The model under review builds one solid part; all positions refer to its coordinate system, in mm. A direction names the side the tool comes from. Give positions to 0.01 mm unless a question says otherwise; leave off trailing zeros. Order: outer loops, then holes, each group sorted by start corner. A loop starts at its lowest first (then second) coordinate and runs counter-clockwise, first axis right, second up.
```python
from build123d import *

# Parameters (mm, degrees)
F1_DEPTH  = 17.5
F2_R      = 2.25021
F2_R_2    = 2.117892
F2_R_3    = 2.141219
F2_R_4    = 1.925027
F2_R_5    = 3.371511
F2_R_6    = 3.105781
F2_R_7    = 1.98861
F2_R_8    = 1.899979
F2_R_9    = 1.912547
F3_DEPTH  = 40
F4_R      = 2.117892
F4_R_2    = 2.25021
F5_DEPTH  = 5
F6_R      = 2.141219
F6_R_2    = 1.925027
F7_DEPTH  = 3
F9_DEPTH  = 3
F10_W     = 16.805832
F10_H     = 44.291496
F10_R     = 3.105781
F10_R_2   = 3.371511
F11_DEPTH = 2


with BuildPart() as f1:
    # F0 (on Front) → F1 (new body)
    with BuildSketch(Plane.XZ):
        Polygon((-29.036315, 123.591392), (-62.036315, 123.591392), (-62.036315, 112.341392), (-79.036315, 112.341392), (-79.036315, 101.091392), (-95.036315, 101.091392), (-95.036315, 56.091392), (-79.036315, 56.091392), (-79.313149, 44.841392), (-62.036315, 44.841392), (-62.036315, 33.591392), (-29.036315, 33.591392), (-29.036315, 58.591392), (-35.036315, 58.591392), (-35.036315, 98.591392), (-29.036315, 98.591392), align=None)
    extrude(amount=F1_DEPTH)

    # F2 (on face) → F3 (cut)
    with BuildSketch(Plane(origin=(-95.036315, 0, 0), x_dir=(0, -1, 0), z_dir=(-1, 0, 0))):
        with Locations((13.294209, 118.739031)):
            Circle(F2_R)
        with Locations((4.177382, 118.739031)):
            Circle(F2_R_2)
        with Locations((4.177382, 106.985271)):
            Circle(F2_R_3)
        with Locations((13.294209, 106.985271)):
            Circle(F2_R_4)
        with Locations((4.177382, 95.644102)):
            Circle(F2_R_5)
        with Locations((4.177382, 84.471688)):
            Circle(F2_R_6)
        with Locations((4.177382, 39.11674)):
            Circle(F2_R_7)
        with Locations((8.744364, 39.11674)):
            Circle(F2_R_8)
        with Locations((13.294209, 39.11674)):
            Circle(F2_R_9)
    extrude(amount=-F3_DEPTH, mode=Mode.SUBTRACT)

    # F4 (on face) → F5 (cut)
    with BuildSketch(Plane(origin=(-62.036315, 0, 0), x_dir=(0, -1, 0), z_dir=(-1, 0, 0))):
        with BuildLine():
            Line((13.491717, 121.922452), (4.209779, 121.922452))
            ThreePointArc((4.209779, 121.922452), (2.088459, 121.043773), (1.209779, 118.922452))
            Line((1.209779, 118.922452), (1.209779, 118.510082))
            ThreePointArc((1.209779, 118.510082), (2.088459, 116.388762), (4.209779, 115.510082))
            Line((4.209779, 115.510082), (13.491717, 115.510082))
            ThreePointArc((13.491717, 115.510082), (15.613037, 116.388762), (16.491717, 118.510082))
            Line((16.491717, 118.510082), (16.491717, 118.922452))
            ThreePointArc((16.491717, 118.922452), (15.613037, 121.043773), (13.491717, 121.922452))
        make_face()
        with Locations((4.177382, 118.739031)):
            Circle(F4_R, mode=Mode.SUBTRACT)
        with Locations((13.294209, 118.739031)):
            Circle(F4_R_2, mode=Mode.SUBTRACT)
    extrude(amount=-F5_DEPTH, mode=Mode.SUBTRACT)

    # F6 (on face) → F7 (cut)
    with BuildSketch(Plane(origin=(-79.036315, 0, 0), x_dir=(0, -1, 0), z_dir=(-1, 0, 0))):
        with BuildLine():
            Line((13.656557, 110.275699), (3.933159, 110.275699))
            ThreePointArc((3.933159, 110.275699), (1.811838, 109.397019), (0.933159, 107.275699))
            Line((0.933159, 107.275699), (0.933159, 106.589088))
            ThreePointArc((0.933159, 106.589088), (1.811838, 104.467767), (3.933159, 103.589088))
            Line((3.933159, 103.589088), (13.656557, 103.589088))
            ThreePointArc((13.656557, 103.589088), (15.777877, 104.467767), (16.656557, 106.589088))
            Line((16.656557, 106.589088), (16.656557, 107.275699))
            ThreePointArc((16.656557, 107.275699), (15.777877, 109.397019), (13.656557, 110.275699))
        make_face()
        with Locations((4.177382, 106.985271)):
            Circle(F6_R, mode=Mode.SUBTRACT)
        with Locations((13.294209, 106.985271)):
            Circle(F6_R_2, mode=Mode.SUBTRACT)
    extrude(amount=-F7_DEPTH, mode=Mode.SUBTRACT)

    # F8 (on face) → F9 (cut)
    with BuildSketch(Plane(origin=(-62.036315, 0, 0), x_dir=(0, -1, 0), z_dir=(-1, 0, 0))):
        with BuildLine():
            ThreePointArc((1.226484, 38.683788), (2.105164, 36.562468), (4.226484, 35.683788))
            Line((4.226484, 35.683788), (13.570151, 35.683788))
            ThreePointArc((13.570151, 35.683788), (15.691471, 36.562468), (16.570151, 38.683788))
            Line((16.570151, 38.683788), (16.570151, 39.214782))
            ThreePointArc((16.570151, 39.214782), (15.691471, 41.336103), (13.570151, 42.214782))
            Line((13.570151, 42.214782), (4.226484, 42.214782))
            ThreePointArc((4.226484, 42.214782), (2.105164, 41.336103), (1.226484, 39.214782))
            Line((1.226484, 39.214782), (1.226484, 38.683788))
        make_face()
    extrude(amount=-F9_DEPTH, mode=Mode.SUBTRACT)

    # F10 (on face) → F11 (cut)
    with BuildSketch(Plane(origin=(-95.036315, 0, 0), x_dir=(0, -1, 0), z_dir=(-1, 0, 0))):
        with Locations((8.686814, 78.51769)):
            Rectangle(F10_W, F10_H)
        with Locations((4.177382, 84.471688)):
            Circle(F10_R, mode=Mode.SUBTRACT)
        with Locations((4.177382, 95.644102)):
            Circle(F10_R_2, mode=Mode.SUBTRACT)
    extrude(amount=-F11_DEPTH, mode=Mode.SUBTRACT)


solid = f1.part
```
Item 1: For faces 4 (the flat face through (-70, -9, 112.341)), 5 (the flat face through (-29.036, -9, 46)), 6 (the cylindrical face through (-57.064, -9.766, 40.719)), list the 3-axis set-ups (+Z, -Z, +X, -X, +Y, -Y) from which the entire face can be reached by the end or side of a thin tool; tool diameter is ignored.
Values found:
face 4: +Z, -X, +Y, -Y
face 5: +Z, -Z, +X, +Y, -Y
face 6: -X
Item 2: For line 1 (Z direction, x = -75.5, y = -4); line 2 (Z direction, x = -65, y = -2); line 3 (Z direction, x = -87, y = -8.5), list the stretches that pass through material, from the lowest coordinate up.
Values found:
line 1: z = 44.84 to 81.37, 87.57 to 92.28, 99.01 to 104.85, 109.12 to 112.34
line 2: z = 44.84 to 82.26, 86.69 to 93.07, 98.22 to 112.34
line 3: z = 56.09 to 101.09
Item 3: Clearance check with flat-ended pins moving along their axes: pin 1 Ø2.5 at (x, y) = (-78, -7) entering from +Z; pin 2 Ø2 at (y, z) = (-10.5, 96) entering from +X; pin 3 Ø5 at (y, z) = (-5.5, 39.5) entering from -X; pin 4 Ø10 at (x, y) = (-65.5, -6.5) entering from +Z. State where each tip first meets the part, or that it passes through.
Values found:
pin 1: stops at z = 112.34
pin 2: stops at x = -35.04
pin 3: stops at x = -59.04
pin 4: stops at z = 123.59
Item 4: Draft analysis for pull direction Z (two halves, no side actions). For faces 1 (the flat face through (-45, -9, 123.591)), 2 (the flat face through (-62, 0, 79)), 3 (the flat face through (-93.036, -9, 79)), state which applies: released by +Z, released by -Z, zero draft, split by the parting line, or undercut.
Values found:
face 1: released by +Z
face 2: zero draft
face 3: undercut
Item 5: Take a section at B-B (z = 74). Give the boundary of the cut face in (x, y), and give its area (3 significant figures).
Values found:
outline: (-95.04, -17.5) - (-35.04, -17.5) - (-35.04, 0) - (-95.04, 0) - (-95.04, -0.28) - (-93.04, -0.28) - (-93.04, -17.09) - (-95.04, -17.09) - close
area: 1,020 mm2
Item 6: Take a section at D-D (x = -77). Give the boundary of the cut face in (y, z), and give its area (3 significant figures).
Values found:
outline: (-17.5, 44.84) - (0, 44.84) - (0, 112.34) - (-17.5, 112.34) - close; hole (-16.66, 106.59) arc R3 ccw to (-13.66, 103.59) - (-3.93, 103.59) arc R3 ccw to (-0.93, 106.59) - (-0.93, 107.28) arc R3 ccw to (-3.93, 110.28) - (-13.66, 110.28) arc R3 ccw to (-16.66, 107.28) - close; hole circle Ø6.74 at (-4.18, 95.64); hole circle Ø6.21 at (-4.18, 84.47)
area: 1,020 mm2
Item 7: Take a section at A-A (x = -64.5). Give the boundary of the cut face in (y, z), and give its area (3 significant figures).
Values found:
outline: (-17.5, 44.84) - (0, 44.84) - (0, 112.34) - (-17.5, 112.34) - close; hole circle Ø3.85 at (-13.29, 106.99); hole circle Ø6.74 at (-4.18, 95.64); hole circle Ø6.21 at (-4.18, 84.47); hole circle Ø4.28 at (-4.18, 106.99)
area: 1,090 mm2
Item 8: Take a section at C-C (x = -84). Give the boundary of the cut face in (y, z).
Values found:
outline: (-17.5, 56.09) - (0, 56.09) - (0, 101.09) - (-17.5, 101.09) - close; hole circle Ø6.74 at (-4.18, 95.64); hole circle Ø6.21 at (-4.18, 84.47)
